CAD build for the part. Positions are in the model's coordinates, mm. Face numbers are marked on the shaded views. Give positions to 0.01 mm unless a question says otherwise; leave off trailing zeros. Order: outer loops, then holes, each group sorted by start corner. A loop starts at its lowest first (then second) coordinate and runs counter-clockwise, first axis right, second up. Notation, with made-up numbers: (66.5, -5) -> (81.5, -5) arc R28 ccw to (81.5, 28) -> close; hole circle Ø8 at (-23, 26). An arc over 180 degrees is marked (long way). Use one line per item in the form item = value. Start each with the question number.
1) Cut at B-B, the plane x = 11. Give the cut face in (y, z).
2) Mould opens along Y. For the marked faces 1, 2, 3 and 4 say: pulls with the +Y half, pulls with the -Y half, needs draft (parallel to the pull), parting line crosses it, or undercut.
3) Cut at D-D, the plane y = 13. Give the cut face in (x, z).
4) Drop flat-ended pins along their axis: P1, Ø4, axis at x = 6, y = 55.5, coming from the +Z side; P2, Ø8, axis at x = 14, z = -85, coming from the -Y side; P3, Ø6, axis at x = 10, y = 44, coming from the -Z side; P4, Ø6, axis at x = 8, y = 38, coming from the +Z side. Give the stop position or say it passes through.
5) Cut at A-A, the plane y = 40. Give the cut face in (x, z), and give its area (3 significant figures).
6) Cut at C-C, the plane y = 63. Give the cut face in (x, z).
7) Probe line 1 (Y direction, x = 9.25, z = -40); line 2 (Z direction, x = 10, y = 41); line 3 (Z direction, x = 23.25, y = 33). List the from-to ranges inside material, lowest first.
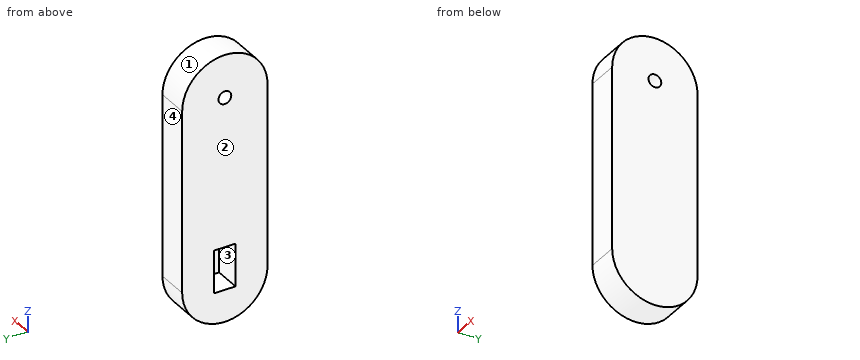
from build123d import *

# Parameters (mm, degrees)
SKETCH2_W               = 250
SKETCH2_H               = 80
BOSS_EXTRUDE1_DEPTH     = 30
SKETCH11_R              = 6
CUT_EXTRUDE2_DEPTH      = 265.196896272
CUT_EXTRUDE_THIN2_DEPTH = 265.196896272
SKETCH15_W              = 40
SKETCH15_H              = 20
CUT_EXTRUDE3_DEPTH      = 25


with BuildPart() as part:
    # Sketch2 → Boss-Extrude1 (new body)
    with BuildSketch(Plane(origin=(0, 0, 0), x_dir=(0, 0, -1), z_dir=(1, 0, 0))):
        with Locations((125, 40)):
            Rectangle(SKETCH2_W, SKETCH2_H)
    extrude(amount=BOSS_EXTRUDE1_DEPTH)

    # Sketch11 → Cut-Extrude2 (cut, through all)
    with BuildSketch(Plane(origin=(30, 0, 0), x_dir=(0, 0, -1), z_dir=(1, 0, 0))):
        with Locations((40, 40)):
            Circle(SKETCH11_R)
    extrude(amount=-CUT_EXTRUDE2_DEPTH, mode=Mode.SUBTRACT)

    # Sketch14 → Cut-Extrude-Thin2 (cut, through all)
    with BuildSketch(Plane.ZY):
        with BuildLine():
            ThreePointArc((-40, 0), (0, 40), (-40, 80))
            Line((-40, 80), (-40, 90))
            ThreePointArc((-40, 90), (10, 40), (-40, -10))
            Line((-40, -10), (-40, 0))
        make_face()
        with BuildLine():
            ThreePointArc((-210, 80), (-250, 40), (-210, 0))
            Line((-210, 0), (-210, -10))
            ThreePointArc((-210, -10), (-260, 40), (-210, 90))
            Line((-210, 90), (-210, 80))
        make_face()
    extrude(amount=-CUT_EXTRUDE_THIN2_DEPTH, mode=Mode.SUBTRACT)


with BuildPart() as cut_extrude_thin2_kept_piece:
    # of the separate pieces the step leaves, the one the design keeps (cut_extrude_thin2_pieces_kept)
    add(part.part.solids().sort_by_distance((0, 0, -40))[0])

    # Sketch15 → Cut-Extrude3 (cut)
    with BuildSketch(Plane.ZY):
        with Locations((-200, 40)):
            Rectangle(SKETCH15_W, SKETCH15_H)
    extrude(amount=-CUT_EXTRUDE3_DEPTH, mode=Mode.SUBTRACT)


solid = cut_extrude_thin2_kept_piece.part
Result:
q1.outline = (0, -210) arc R40 ccw to (80, -210) -> (80, -40) arc R40 ccw to (0, -40) -> close; hole (30, -220) -> (50, -220) -> (50, -180) -> (30, -180) -> close; hole circle Ø12 at (40, -40)
q2.face_1 = parting line crosses it
q2.face_2 = needs draft
q2.face_3 = undercut
q2.face_4 = pulls with the +Y half
q3.outline = (0, -239.51) -> (30, -239.51) -> (30, -10.49) -> (0, -10.49) -> close
q4.P1 = -2.35
q4.P2 = 0
q4.P3 = -249.99
q4.P4 = 0
q5.outline = (0, -250) -> (30, -250) -> (30, -46) -> (0, -46) -> (0, -180) -> (25, -180) -> (25, -220) -> (0, -220) -> close; (0, -34) -> (30, -34) -> (30, 0) -> (0, 0) -> close
q5.area = 6,140 mm²
q6.outline = (0, -242.73) -> (30, -242.73) -> (30, -7.27) -> (0, -7.27) -> close
q7.line_1 = 0 to 34, 46 to 80
q7.line_2 = -249.99 to -220, -180 to -45.92, -34.08 to -0.01
q7.line_3 = -249.38 to -220, -180 to -0.62
